Build history of the part. All positions in model axes, mm. A direction names the side the tool comes from. Give positions to 0.01 mm unless a question says otherwise; leave off trailing zeros. Order: outer loops, then holes, each group sorted by start corner. A loop starts at its lowest first (then second) coordinate and runs counter-clockwise, first axis right, second up. Notation, with made-up numbers: (84.5, -0.75) -> (117.5, -0.75) arc R26 ccw to (117.5, 26.25) -> close; hole circle Ø11 at (86, -17.5). An arc over 180 degrees is marked (long way). One line per item, written item: value. Start each with the question number.
(1) Saw through at B-B on z = 0. Give the cut face in (x, y) (3 decimals).
(2) Saw through at C-C on y = -2.75. Give the cut face in (x, z) (3 decimals), plus the area to 3 significant figures.
(3) Pin check, flat tips, straight feed: pin 1 (1.3 mm diameter, centred on y = 1.5, z = -6, fed in from +X) (3 decimals); pin 2 (2.5 mm diameter, centred on x = -2.5, z = -0.5, fed in from +Y); pin 3 (2.5 mm diameter, centred on x = 5.5, y = 1, fed in from -Z). Stop position of each tip, or through.
(4) Two-plate mould, pull along X, no slides. Class faces 6 (the flat face through (6.55, 0, 0)), 7 (the flat face through (0, 0, -8.1)), 8 (the flat face through (0.3, 2, 0)): +X half, -X half, draft (parallel to the pull), parting line (faces both ways), or undercut.
(5) Saw through at A-A on z = -5.2. Give the cut face in (x, y) (3 decimals), plus the area to 3 significant figures.
(6) Saw through at D-D on x = 4.25. Give the cut face in (y, z), plus the area to 3 significant figures.
(7) Probe line 1 (X direction, y = -3.35, z = 0) (3 decimals); line 2 (Z direction, x = 0.5, y = -0.5); line 3 (X direction, y = 1.25, z = 0.75). List the from-to ranges inside material, lowest first.
(8) Which spindle directions (+Z, -Z, +X, -X, +Y, -Y) get a long thin tool onto all of the face, cutting with end or side? Do faces 1 (the cylindrical face through (1.53, -3.32, -4.45)), 2 (the flat face through (-3.425, 0, -6)), 3 (the flat face through (3, 2, -2.3)), 4 (the flat face through (5, 0, -2.9)), 5 (the flat face through (0, 0, 2.9)). Say none if no direction does.
```python
from build123d import *

# Parameters (mm, degrees)
SKETCH1_W               = 13.1
SKETCH1_H               = 5.8
BOSS_EXTRUDE1_DEPTH     = 5
SKETCH10_W              = 5.65
SKETCH10_H              = 4.6
CUT_EXTRUDE7_DEPTH      = 6.6
CUT_EXTRUDE6_DEPTH      = 9.735702605
CUT_EXTRUDE6_DEPTH_BACK = 9.735702605
SKETCH9_R               = 0.75
BOSS_EXTRUDE2_START     = -5
BOSS_EXTRUDE2_DEPTH     = 10
SKETCH12_W              = 5.65
SKETCH12_H              = 4.6
SKETCH12_R              = 0.75
BOSS_EXTRUDE3_DEPTH     = 3.4
FILETE1_R               = 0.5
FILETE2_R               = 0.1


with BuildPart() as part:
    # Sketch1 → Boss-Extrude1 (new, symmetric)
    with BuildSketch(Plane(origin=(0, 0, 0), x_dir=(1, 0, 0), z_dir=(0, 1, 0))):
        Rectangle(SKETCH1_W, SKETCH1_H)
    extrude(amount=BOSS_EXTRUDE1_DEPTH, both=True)

    # Sketch10 → Cut-Extrude7 (cut)
    with BuildSketch(Plane(origin=(0, 5, 0), x_dir=(1, 0, 0), z_dir=(0, 1, 0))):
        with Locations((-3.125, 0)):
            Rectangle(SKETCH10_W, SKETCH10_H)
        with Locations((3.125, 0)):
            Rectangle(SKETCH10_W, SKETCH10_H)
    extrude(amount=-CUT_EXTRUDE7_DEPTH, mode=Mode.SUBTRACT)

    # Sketch9 → Cut-Extrude6 (cut, two sides: drawn at the far end of the back side and taken through both)
    with BuildSketch(Plane(origin=(0, 0, 0), x_dir=(1, 0, 0), z_dir=(0, 1, 0)).offset(-CUT_EXTRUDE6_DEPTH_BACK)):
        with Locations(Location((-4.625, 0, 0), (0, 0, 270))):
            Circle(SKETCH9_R)
        with Locations(Location((-1.625, 0, 0), (0, 0, 270))):
            Circle(SKETCH9_R)
        with Locations(Location((1.625, 0, 0), (0, 0, 270))):
            Circle(SKETCH9_R)
        with Locations(Location((4.625, 0, 0), (0, 0, 270))):
            Circle(SKETCH9_R)
    extrude(amount=CUT_EXTRUDE6_DEPTH + CUT_EXTRUDE6_DEPTH_BACK, mode=Mode.SUBTRACT)

    # Sketch11 → Boss-Extrude2 (add)
    with BuildSketch(Plane(origin=(0, 0, 0), x_dir=(1, 0, 0), z_dir=(0, 1, 0)).offset(BOSS_EXTRUDE2_START)):
        Polygon((-3.425, 8.1), (-3.425, 2.9), (-2.825, 2.9), (-2.825, 7.5), (2.825, 7.5), (2.825, 2.9), (3.425, 2.9), (3.425, 8.1), align=None)
    extrude(amount=BOSS_EXTRUDE2_DEPTH)

    # Sketch12 → Boss-Extrude3 (add)
    with BuildSketch(Plane.XZ.offset(5)):
        with Locations((0, -5.2)):
            Rectangle(SKETCH12_W, SKETCH12_H)
        with Locations(Location((-1.5, -5.2, 0), (0, 0, 270))):
            Circle(SKETCH12_R, mode=Mode.SUBTRACT)
        with Locations(Location((1.5, -5.2, 0), (0, 0, 270))):
            Circle(SKETCH12_R, mode=Mode.SUBTRACT)
    extrude(amount=-BOSS_EXTRUDE3_DEPTH)

    # Filete1
    filete1_edges = [part.edges().sort_by_distance(p)[0] for p in [
        (-6.55, 0, -2.9),
        (-3.425, 0, -2.9),
        (-3.425, 0, -8.1),
        (3.425, 0, -8.1),
        (6.55, 0, -2.9),
        (3.425, 0, -2.9),
        (6.55, 0, 2.9),
        (-6.55, 0, 2.9),
    ]]
    fillet(filete1_edges, radius=FILETE1_R)

    # Filete2
    filete2_edges = [part.edges().sort_by_distance(p)[0] for p in [
        (-5.95, 1.7, 2.3),
        (-5.95, 1.7, -2.3),
        (-0.3, 1.7, -2.3),
        (-0.3, 1.7, 2.3),
        (5.95, 1.7, 2.3),
        (0.3, 1.7, 2.3),
        (0.3, 1.7, -2.3),
        (5.95, 1.7, -2.3),
        (2.825, 1.7, -7.5),
        (-2.825, 1.7, -7.5),
        (-2.825, 1.7, -2.9),
        (2.825, 1.7, -2.9),
    ]]
    fillet(filete2_edges, radius=FILETE2_R)


solid = part.part
```
Results below:
1. outline: (-6.55, -5) -> (-5.375, -5) -> (-5.375, -1.6) -> (-5.95, -1.6) -> (-5.95, 5) -> (-6.55, 5) -> close; (-3.875, -5) -> (-2.375, -5) -> (-2.375, -1.6) -> (-3.875, -1.6) -> close; (-0.875, -5) -> (0.875, -5) -> (0.875, -1.6) -> (0.3, -1.6) -> (0.3, 5) -> (-0.3, 5) -> (-0.3, -1.6) -> (-0.875, -1.6) -> close; (2.375, -5) -> (3.875, -5) -> (3.875, -1.6) -> (2.375, -1.6) -> close; (5.375, -5) -> (6.55, -5) -> (6.55, 5) -> (5.95, 5) -> (5.95, -1.6) -> (5.375, -1.6) -> close
2. outline: (-6.55, -2.4) arc R0.5 ccw to (-6.05, -2.9) -> (-3.925, -2.9) arc R0.5 cw to (-3.425, -3.4) -> (-3.425, -7.6) arc R0.5 ccw to (-2.925, -8.1) -> (2.925, -8.1) arc R0.5 ccw to (3.425, -7.6) -> (3.425, -3.4) arc R0.5 cw to (3.925, -2.9) -> (6.05, -2.9) arc R0.5 ccw to (6.55, -2.4) -> (6.55, 2.4) arc R0.5 ccw to (6.05, 2.9) -> (-6.05, 2.9) arc R0.5 ccw to (-6.55, 2.4) -> close; hole circle Ø1.5 at (-4.625, 0); hole circle Ø1.5 at (-1.625, 0); hole circle Ø1.5 at (-1.5, -5.2); hole circle Ø1.5 at (1.5, -5.2); hole circle Ø1.5 at (1.625, 0); hole circle Ø1.5 at (4.625, 0)
2. area: 101 mm²
3. pin 1: stops at x = 3.425
3. pin 2: stops at y = -1.6
3. pin 3: stops at z = -2.9
4. face 6: +X half
4. face 7: draft
4. face 8: undercut
5. outline: (-3.425, -5) -> (-2.25, -5) -> (-2.25, -1.6) -> (-2.825, -1.6) -> (-2.825, 5) -> (-3.425, 5) -> close; (-0.75, -5) -> (0.75, -5) -> (0.75, -1.6) -> (-0.75, -1.6) -> close; (2.25, -5) -> (3.425, -5) -> (3.425, 5) -> (2.825, 5) -> (2.825, -1.6) -> (2.25, -1.6) -> close
5. area: 21.0 mm²
6. outline: (-5, -2.9) -> (5, -2.9) -> (5, -2.3) -> (-1.6, -2.3) -> (-1.6, -0.65) -> (-5, -0.65) -> close; (-5, 0.65) -> (-1.6, 0.65) -> (-1.6, 2.3) -> (5, 2.3) -> (5, 2.9) -> (-5, 2.9) -> close
6. area: 23.2 mm²
7. line 1: x = -6.55 to -5.375, -3.875 to -2.375, -0.875 to 0.875, 2.375 to 3.875, 5.375 to 6.55
7. line 2: z = -8.1 to -7.5, -2.9 to -2.3, 2.3 to 2.9
7. line 3: x = -6.55 to -5.95, -0.3 to 0.3, 5.95 to 6.55
8. face 1: +Y, -Y
8. face 2: -Z, -X, +Y, -Y
8. face 3: +Y
8. face 4: -Z, +X, +Y, -Y
8. face 5: +Z, +X, -X, +Y, -Y
